Autodesk Fusion 360 part; units mm, degrees
sketch "Sketch1" plane through (0, 0, 0) normal (0, 0, 1) x (1, 0, 0)
  line L0 (0, 0) -> (152.4, 0)
  line L1 (152.4, 0) -> (152.4, -101.6)
  line L2 (152.4, -101.6) -> (0, -101.6)
  line L3 (0, -101.6) -> (0, 0)
  dimension "d1" = 152.4
  dimension "d2" = 101.6
extrude "Extrude1" add sketch "Sketch1" along normal blind 31.75
fillet "Fillet1" radius 12.7 4 edges at (0, -101.6, 15.875) (152.4, -101.6, 15.875) (152.4, 0, 15.875) (0, 0, 15.875)
sketch "Sketch2" plane through (0, 0, 31.75) normal (0, 0, 1) x (-1, 0, 0)
  arc A0 (-12.7, 0) -> (0, 12.7) centre (-12.7, 12.7) ccw
  line L0 (0, 12.7) -> (0, 88.9)
  arc A1 (0, 88.9) -> (-12.7, 101.6) centre (-12.7, 88.9) ccw
  line L1 (-12.7, 101.6) -> (-139.7, 101.6)
  arc A2 (-139.7, 101.6) -> (-152.4, 88.9) centre (-139.7, 88.9) ccw
  line L2 (-152.4, 88.9) -> (-152.4, 12.7)
  arc A3 (-152.4, 12.7) -> (-139.7, 0) centre (-139.7, 12.7) ccw
  line L3 (-139.7, 0) -> (-12.7, 0)
  line L4 (-7.62, 12.7) -> (-7.62, 88.9)
  arc A4 (-7.62, 88.9) -> (-12.7, 93.98) centre (-12.7, 88.9) ccw
  line L5 (-12.7, 93.98) -> (-139.7, 93.98)
  arc A5 (-139.7, 93.98) -> (-144.78, 88.9) centre (-139.7, 88.9) ccw
  line L6 (-144.78, 88.9) -> (-144.78, 12.7)
  arc A6 (-144.78, 12.7) -> (-139.7, 7.62) centre (-139.7, 12.7) ccw
  line L7 (-139.7, 7.62) -> (-12.7, 7.62)
  arc A7 (-12.7, 7.62) -> (-7.62, 12.7) centre (-12.7, 12.7) ccw
  circle A8 centre (-12.7, 12.7) radius 12.7
  circle A9 centre (-139.7, 12.7) radius 12.7
  circle A10 centre (-139.7, 88.9) radius 12.7
  circle A11 centre (-12.7, 88.9) radius 12.7
  dimension "d7" = -7.62
  dimension "d8" = 25.4
  dimension "d9" = 25.4
  dimension "d10" = 25.4
  dimension "d11" = 25.4
extrude "Extrude2" cut sketch "Sketch2" against normal blind 25.4 contours L4 L5 L6 L7 A8 A9 A10 A11
fillet "Fillet2" radius 5.08 8 edges at (144.78, -24.3397, 19.05) (128.0603, -7.62, 19.05) (24.3397, -7.62, 19.05) (7.62, -24.3397, 19.05) (24.3397, -93.98, 19.05) (7.62, -77.2603, 19.05) (144.78, -77.2603, 19.05) (128.0603, -93.98, 19.05)
sketch "Sketch3" plane through (0, 0, 31.75) normal (0, 0, 1) x (-1, 0, 0)
  line L0 (-121.92, 93.98) -> (-30.48, 93.98)
  arc A0 (-25.4, 88.9) -> (-30.48, 93.98) centre (-30.48, 88.9) ccw
  arc A1 (-25.4, 88.9) -> (-12.7, 76.2) centre (-12.7, 88.9) ccw
  arc A2 (-7.62, 71.12) -> (-12.7, 76.2) centre (-12.7, 71.12) ccw
  line L1 (-7.62, 71.12) -> (-7.62, 30.48)
  arc A3 (-12.7, 25.4) -> (-7.62, 30.48) centre (-12.7, 30.48) ccw
  arc A4 (-12.7, 25.4) -> (-25.4, 12.7) centre (-12.7, 12.7) ccw
  arc A5 (-30.48, 7.62) -> (-25.4, 12.7) centre (-30.48, 12.7) ccw
  line L2 (-30.48, 7.62) -> (-121.92, 7.62)
  arc A6 (-127, 12.7) -> (-121.92, 7.62) centre (-121.92, 12.7) ccw
  arc A7 (-127, 12.7) -> (-139.7, 25.4) centre (-139.7, 12.7) ccw
  arc A8 (-144.78, 30.48) -> (-139.7, 25.4) centre (-139.7, 30.48) ccw
  line L3 (-144.78, 30.48) -> (-144.78, 71.12)
  arc A9 (-139.7, 76.2) -> (-144.78, 71.12) centre (-139.7, 71.12) ccw
  arc A10 (-139.7, 76.2) -> (-127, 88.9) centre (-139.7, 88.9) ccw
  arc A11 (-121.92, 93.98) -> (-127, 88.9) centre (-121.92, 88.9) ccw
  arc A12 (-12.7, 0) -> (0, 12.7) centre (-12.7, 12.7) ccw
  line L4 (0, 12.7) -> (0, 88.9)
  arc A13 (0, 88.9) -> (-12.7, 101.6) centre (-12.7, 88.9) ccw
  line L5 (-12.7, 101.6) -> (-139.7, 101.6)
  arc A14 (-139.7, 101.6) -> (-152.4, 88.9) centre (-139.7, 88.9) ccw
  line L6 (-152.4, 88.9) -> (-152.4, 12.7)
  arc A15 (-152.4, 12.7) -> (-139.7, 0) centre (-139.7, 12.7) ccw
  line L7 (-139.7, 0) -> (-12.7, 0)
  point P0 (-12.7, 88.9)
  point P1 (-12.7, 12.7)
  point P2 (-139.7, 12.7)
  point P3 (-139.7, 88.9)
hole "Hole1" at (12.7, -12.7, 31.75) at (139.7, -88.9, 31.75) at (139.7, -12.7, 31.75) at (12.7, -88.9, 31.75) direction (0, 0, -1) diameter 9.906 end through all counterbore diameter 14.224 counterbore depth 10.16
sketch "Sketch4" plane through (0, -101.6, 0) normal (0, -1, 0) x (1, 0, 0)
  line L0 (139.7, 0) -> (139.7, 31.75)
  line L1 (139.7, 31.75) -> (12.7, 31.75)
  line L2 (12.7, 31.75) -> (12.7, 0)
  line L3 (12.7, 0) -> (139.7, 0)
  line L4 (57.15, 12.7) -> (95.25, 12.7)
  arc A0 (95.25, 12.7) -> (95.25, 25.4) centre (95.25, 19.05) ccw
  line L5 (95.25, 25.4) -> (57.15, 25.4)
  arc A1 (57.15, 25.4) -> (57.15, 12.7) centre (57.15, 19.05) ccw
  line L6 (50.8, 19.05) -> (101.6, 19.05) construction
  line L7 (0, 31.75) -> (0, 0)
  circle A2 centre (57.15, 19.05) radius 3.175
  circle A3 centre (95.25, 19.05) radius 3.175
  point P0 (76.2, 19.05)
  dimension "d21" = 12.7
  dimension "d22" = 76.2
  dimension "d23" = 12.7
  dimension "d24" = 6.35
  dimension "d25" = 6.35
extrude "Extrude4" cut sketch "Sketch4" against normal blind 5.08 contours L4 A0 L5 A1
extrude "Extrude3" cut sketch "Sketch4" against normal through all contours A2 | A3
sketch "Sketch6" plane through (0, 0, 0) normal (0, 1, 0) x (-1, 0, 0)
  circle A0 centre (-57.15, 19.05) radius 3.175
  circle A1 centre (-95.25, 19.05) radius 3.175
  line L0 (-12.7, 0) -> (-12.7, 31.75)
  line L1 (-12.7, 31.75) -> (-139.7, 31.75)
  line L2 (-139.7, 31.75) -> (-139.7, 0)
  line L3 (-139.7, 0) -> (-12.7, 0)
  line L4 (-57.15, 25.4) -> (-95.25, 25.4)
  arc A2 (-95.25, 25.4) -> (-95.25, 12.7) centre (-95.25, 19.05) ccw
  line L5 (-95.25, 12.7) -> (-57.15, 12.7)
  arc A3 (-57.15, 12.7) -> (-57.15, 25.4) centre (-57.15, 19.05) ccw
  line L6 (-57.15, 19.05) -> (-95.25, 19.05) construction
  dimension "d29" = 12.7
extrude "Extrude5" cut sketch "Sketch6" against normal blind 5.08 contours L4 A2 L5 A3
equation "d25 = d24"
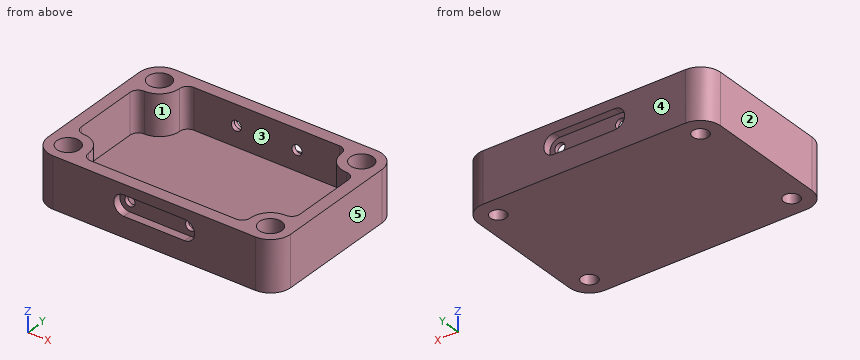
Check sheet for the modelled part. Datum: model origin and axes. Units: mm. Face numbers are marked on the shaded views. A direction names the side the tool comes from. Give positions to 0.01 mm unless a question says otherwise; leave off trailing zeros. Write each loop counter-clockwise with the first axis right and the second up, starting at its lowest first coordinate (ties: lowest second). Pieces come first, ordered by that corner, then holes. Notation, with made-up numbers: M 13.25,80.25 L 38.25,80.25 A24 ccw 38.25,110.25 Z; hole C 49,6 d2. An arc over 180 degrees is marked long. Use one line per item in the form item = value.
(1) Section check B-B on x = 70.5. Record the boundary of the cut face in (y, z), plus the area to 3 significant figures.
Answer block:
outline = M -101.6,0 L 0,0 L 0,12.7 L -5.08,12.7 L -5.08,25.4 L 0,25.4 L 0,31.75 L -7.62,31.75 L -7.62,6.35 L -93.98,6.35 L -93.98,31.75 L -101.6,31.75 L -101.6,25.4 L -96.52,25.4 L -96.52,12.7 L -101.6,12.7 Z
area = 903 mm2
(2) Depth check by flat-ended pin: P1, Ø8, axis at x = 139.7, y = -88.9, coming from the +Z side; P2, Ø2, axis at x = 122.5, y = -76, coming from the +Z side; P3, Ø8.5, axis at x = 95.25, z = 19.05, coming from the -Y side. Enter the tip coordinate at first touch or a pass-through.
Answer block:
P1 = through
P2 = 6.35
P3 = -96.52
(3) Section check C-C on z = 19.05. State how many separate pieces and enclosed holes the cut face has, plus the area to 3 significant figures.
Answer block:
separate_pieces = 4
enclosed_holes = 4
area = 3,780 mm2
(4) Section check D-D on y = -47. Record the boundary of the cut face in (x, z), plus the area to 3 significant figures.
Answer block:
outline = M 0,0 L 152.4,0 L 152.4,31.75 L 144.78,31.75 L 144.78,6.35 L 7.62,6.35 L 7.62,31.75 L 0,31.75 Z
area = 1,350 mm2
(5) Material ranges on line 1 along Y through (x, z) = (12.7, 6); line 2 along Y through (x, z) = (12.7, 25.75); line 3 along Y through (x, z) = (12.7, 13), recorded low to high.
Answer block:
line_1 = -101.6 to -93.85, -83.95 to -17.65, -7.75 to 0
line_2 = -101.6 to -96.01, -81.79 to -76.2, -25.4 to -19.81, -5.59 to 0
line_3 = -101.6 to -93.85, -83.95 to -76.2, -25.4 to -17.65, -7.75 to 0
(6) Tool access check on the marked faces 1 and 2. Record the directions out of +Z, -Z, +X, -X, +Y, -Y that give a thin tool (end or side, any length) a straight path to the whole face; none if there is none.
Answer block:
face_1 = +Z
face_2 = +Z, -Z, -X, +Y, -Y
(7) Draft check along Y on the marked faces 3, 4 and 5. Enter one of: pulls with the +Y half, pulls with the -Y half, needs draft (parallel to the pull), parting line crosses it, or undercut.
Answer block:
face_3 = undercut
face_4 = pulls with the +Y half
face_5 = needs draft
(8) Section check A-A on z = 10.5. Record the boundary of the cut face in (x, y).
Answer block:
outline = M 0,-88.9 A12.7 ccw 12.7,-101.6 L 139.7,-101.6 A12.7 ccw 152.4,-88.9 L 152.4,-12.7 A12.7 ccw 139.7,0 L 12.7,0 A12.7 ccw 0,-12.7 Z; hole M 7.62,-71.12 A5.08 ccw 12.7,-76.2 A12.7 cw 25.4,-88.9 A5.08 ccw 30.48,-93.98 L 121.92,-93.98 A5.08 ccw 127,-88.9 A12.7 cw 139.7,-76.2 A5.08 ccw 144.78,-71.12 L 144.78,-30.48 A5.08 ccw 139.7,-25.4 A12.7 cw 127,-12.7 A5.08 ccw 121.92,-7.62 L 30.48,-7.62 A5.08 ccw 25.4,-12.7 A12.7 cw 12.7,-25.4 A5.08 ccw 7.62,-30.48 Z; hole C 12.7,-88.9 d9.91; hole C 12.7,-12.7 d9.91; hole C 139.7,-88.9 d9.91; hole C 139.7,-12.7 d9.91
